Could you check a few things on this drawing? It's one solid part, dimensions in mm from its lowest x, y, z. Coordinates: 2 decimals unless noted, no trailing zeros. Loops run counter-clockwise (first coordinate to the right, second up) from the corner with the lowest first, then second, coordinate; pieces in that order, holes last.
1) If I drill on line 1 along Y through (x, z) = (44.45, 0.3); line 2 along Y through (x, z) = (46, 1.05), over which ranges is the centre line in solid material (lowest first)?
2) Imagine slicing it at D-D on z = 0.65. Please give me the cut outline in (x, y), plus the area to 3 significant figures.
3) Imagine slicing it at B-B on x = 25.4. Please give me the cut outline in (y, z), plus the area to 3 significant figures.
4) Imagine slicing it at A-A on y = 44.45. Please give me the cut outline in (x, z), plus the area to 3 significant figures.
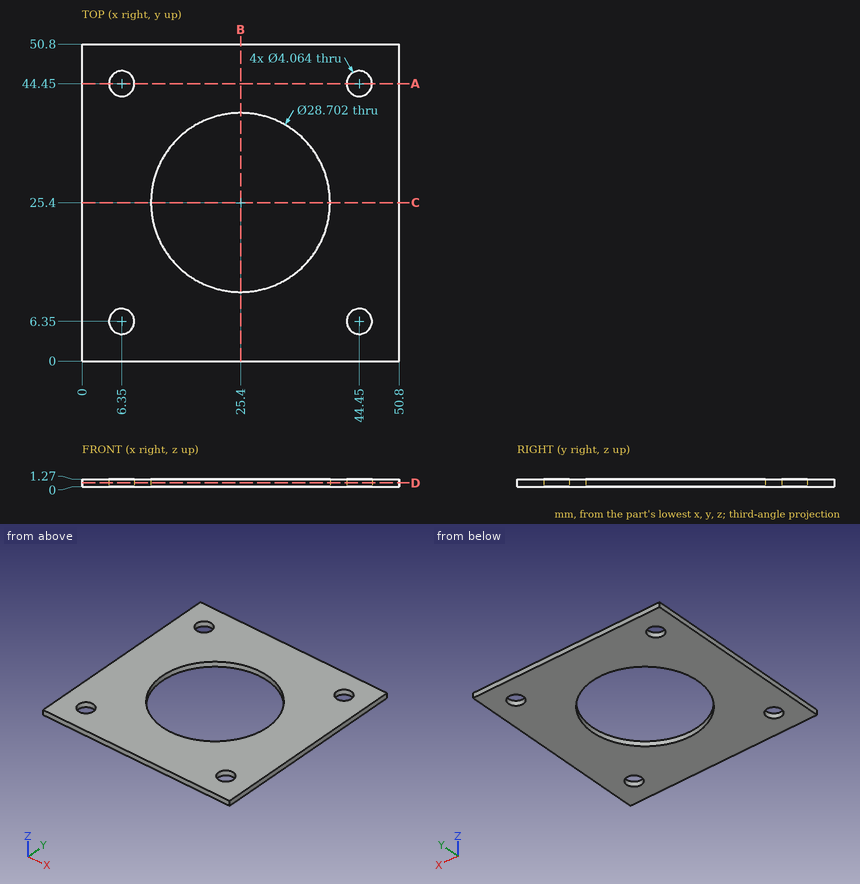
Filled in:
1. line 1: y = 0 to 4.32, 8.38 to 42.42, 46.48 to 50.8
1. line 2: y = 0 to 5.04, 7.66 to 43.14, 45.76 to 50.8
2. outline: (0, 0) - (50.8, 0) - (50.8, 50.8) - (0, 50.8) - close; hole circle Ø4.06 at (6.35, 6.35); hole circle Ø4.06 at (6.35, 44.45); hole circle Ø28.7 at (25.4, 25.4); hole circle Ø4.06 at (44.45, 6.35); hole circle Ø4.06 at (44.45, 44.45)
2. area: 1,880 mm2
3. outline: (0, 0) - (11.05, 0) - (11.05, 1.27) - (0, 1.27) - close; (39.75, 0) - (50.8, 0) - (50.8, 1.27) - (39.75, 1.27) - close
3. area: 28.1 mm2
4. outline: (0, 0) - (4.32, 0) - (4.32, 1.27) - (0, 1.27) - close; (8.38, 0) - (42.42, 0) - (42.42, 1.27) - (8.38, 1.27) - close; (46.48, 0) - (50.8, 0) - (50.8, 1.27) - (46.48, 1.27) - close
4. area: 54.2 mm2
